Part print with two shaded views. Sizes in mm from the minimum x, y, z corner. Coordinates: 2 decimals unless noted, no trailing zeros. Write each loop counter-clockwise with the first axis right and the second up, starting at its lowest first coordinate (ties: lowest second). Pieces come first, ordered by that corner, then holes.
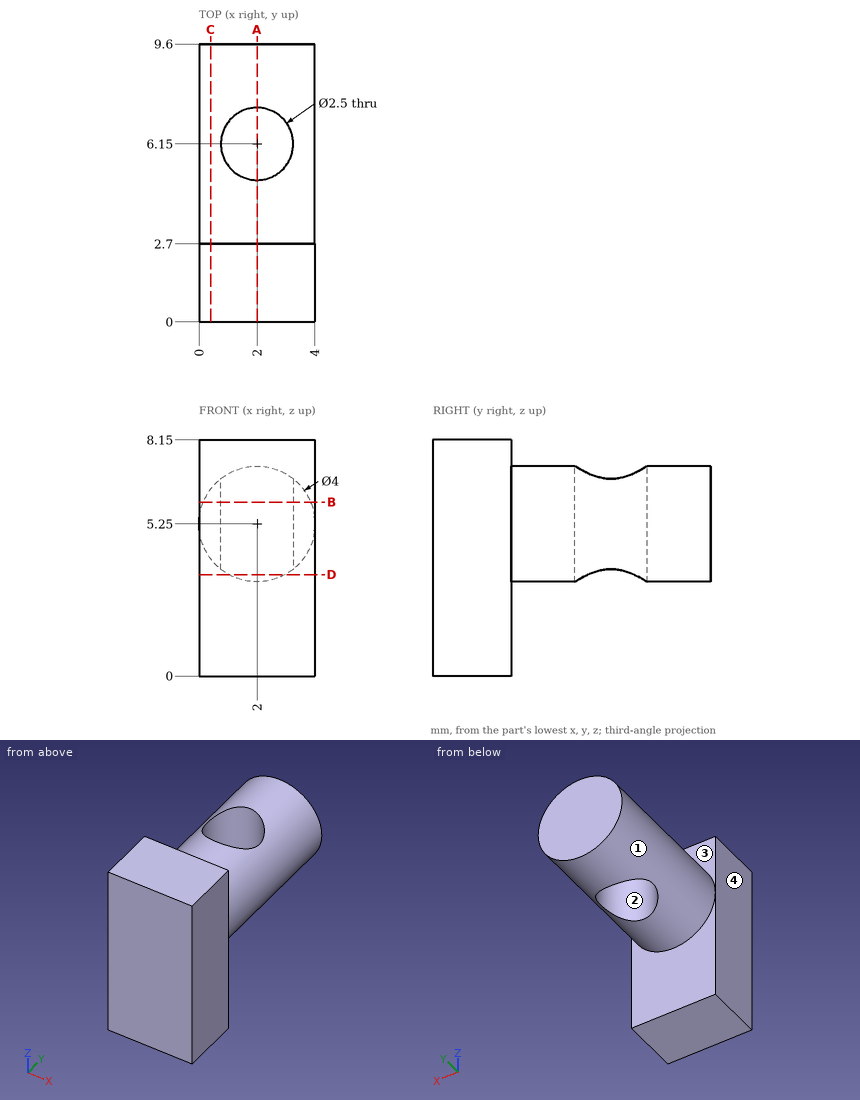
(1) Slice it at A-A, the plane x = 2. List the corners of the cut face in (y, z), and give its area (3 significant figures).
(2) Slice it at C-C, the plane x = 0.4. List the corners of the cut face in (y, z), and give its area (3 significant figures).
(3) Probe L1, parallel to Y at x = 2, z = 5; L2, parallel to X at y = 6.15, z = 5.3; L3, parallel to Y at x = 1.3, z = 6.25. List the from-to ranges inside material, lowest first.
(4) Flat gauge pins, fed straight in: P1, Ø2, axis at x = 2, y = 6.15, coming from the -Z side; P2, Ø1.2, axis at x = 2, z = 2, coming from the +Y side; P3, Ø1, axis at x = 1.5, y = 8, coming from the +Z side; P4, Ø3, axis at y = 7, z = 2.5, coming from the -X side. Where does each tip first touch, or does it go through?
(5) Slice it at D-D, the plane z = 3.5. List the corners of the cut face in (x, y).
(6) Slice it at B-B, the plane z = 6. List the corners of the cut face in (x, y).
(7) Two-plate mould, pull along X, no slides. Class the marked faces 1, 2, 3 and 4: pulls with the +X half, pulls with the -X half, needs draft (parallel to the pull), parting line crosses it, or undercut.
Results:
1. outline: (0, 0) - (2.7, 0) - (2.7, 3.25) - (4.9, 3.25) - (4.9, 7.25) - (2.7, 7.25) - (2.7, 8.15) - (0, 8.15) - close; (7.4, 3.25) - (9.6, 3.25) - (9.6, 7.25) - (7.4, 7.25) - close
1. area: 39.6 mm2
2. outline: (0, 0) - (2.7, 0) - (2.7, 4.05) - (9.6, 4.05) - (9.6, 6.45) - (2.7, 6.45) - (2.7, 8.15) - (0, 8.15) - close
2. area: 38.6 mm2
3. L1: y = 0 to 4.9, 7.4 to 9.6
3. L2: x = 0 to 0.75, 3.25 to 4
3. L3: y = 0 to 5.11, 7.19 to 9.6
4. P1: passes through
4. P2: stops at y = 2.7
4. P3: stops at z = 7.25
4. P4: stops at x = 0.44
5. outline: (0, 0) - (4, 0) - (4, 2.7) - (2.97, 2.7) - (2.97, 5.36) arc R1.25 cw to (1.03, 5.36) - (1.03, 2.7) - (0, 2.7) - close; (1.03, 6.94) arc R1.25 cw to (2.97, 6.94) - (2.97, 9.6) - (1.03, 9.6) - close
6. outline: (0, 0) - (4, 0) - (4, 2.7) - (3.85, 2.7) - (3.85, 9.6) - (0.15, 9.6) - (0.15, 2.7) - (0, 2.7) - close; hole circle Ø2.5 at (2, 6.15)
7. face 1: parting line crosses it
7. face 2: undercut
7. face 3: needs draft
7. face 4: pulls with the -X half
